```python
from build123d import *

# Parameters (mm, degrees)
SKETCH_W     = 32
SKETCH_H     = 17
PAD_DEPTH    = 1.5
SKETCH001_W  = 6
SKETCH001_H  = 6
PAD001_DEPTH = 2
SKETCH002_R  = 2.710161
PAD002_DEPTH = 7
SKETCH003_W  = 20
SKETCH003_H  = 12
PAD003_DEPTH = 4


with BuildPart() as part:
    # Sketch → Pad (new body)
    with BuildSketch(Plane.XZ):
        with Locations((16, 8.5)):
            Rectangle(SKETCH_W, SKETCH_H)
    extrude(amount=PAD_DEPTH)

    # Sketch001 (on Face4 of Pad) → Pad001 (join)
    with BuildSketch(Plane(origin=(0, 0, 0), x_dir=(0, 0, -1), z_dir=(-1, 0, 0))):
        with Locations((-8.5, 1)):
            Rectangle(SKETCH001_W, SKETCH001_H)
    extrude(amount=PAD001_DEPTH)

    # Sketch002 (on Face13 of Pad001) → Pad002 (join)
    with BuildSketch(Plane(origin=(-2, 0, 0), x_dir=(0, 0, -1), z_dir=(-1, 0, 0))):
        with Locations((-8.5, 1)):
            Circle(SKETCH002_R)
    extrude(amount=PAD002_DEPTH)

    # Sketch003 (on Face5 of Pad002) → Pad003 (join)
    with BuildSketch(Plane.XZ.offset(1.5)):
        with Locations((40, 9)):
            Rectangle(SKETCH003_W, SKETCH003_H)
    extrude(amount=PAD003_DEPTH)


solid = part.part
```
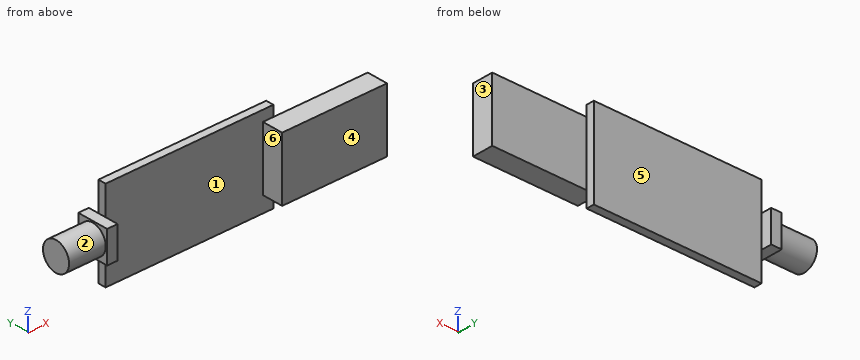
Source: CAD feature listing. Evaluate the final solid. Frame: model axes, mm. Face numbers are marked on the shaded views. A direction names the side the tool comes from. Round coordinates to 2 decimals unless told otherwise and drop trailing zeros. Loops run counter-clockwise (first coordinate to the right, second up) from the corner with the lowest first, then second, coordinate; pieces in that order, holes last. Notation, with made-up numbers: (69, -35.5) - (104, -35.5) arc R21 ccw to (104, -17.5) - close; hole circle Ø2 at (20, 52). An arc over 180 degrees is marked (long way). Use CSV: the item, a comma, the result in double quotes.
Q1. Section query A-A, the plane y = -1. Output: boundary loops of the cut face in (x, z), then the cut area to 3 significant figures.
Reported:
outline,"(-9, 5.79) - (-2, 5.79) - (-2, 5.5) - (0, 5.5) - (0, 0) - (32, 0) - (32, 17) - (0, 17) - (0, 11.5) - (-2, 11.5) - (-2, 11.21) - (-9, 11.21) - close"
area,"594 mm^2"
Q2. Mould query, pull axis X, two halves, no side actions, for the marked faces 1, 2 and 3. Classes: pulls with the +X half, pulls with the -X half, needs draft (parallel to the pull), parting line crosses it, or undercut.
Reported:
face 1,"undercut"
face 2,"needs draft"
face 3,"pulls with the +X half"
Q3. Section query D-D, the plane z = 8.5. Output: boundary loops of the cut face in (x, y), then the cut area to 3 significant figures.
Reported:
outline,"(-9, -3.71) - (-2, -3.71) - (-2, -4) - (0, -4) - (0, -1.5) - (30, -1.5) - (30, -5.5) - (50, -5.5) - (50, -1.5) - (32, -1.5) - (32, 0) - (0, 0) - (0, 2) - (-2, 2) - (-2, 1.71) - (-9, 1.71) - close"
area,"178 mm^2"
Q4. Pin query (flat end, axial travel): pin 1 Ø5 at (x, z) = (9.5, 6.5) entering from +Y; pin 2 Ø4.5 at (x, y) = (41, -2.5) entering from -Z; pin 3 Ø1.2 at (x, y) = (42.5, -3.5) entering from +Z; pin 4 Ø1.5 at (x, y) = (37.5, 1) entering from +Z. Return the tip coordinate at first contact, or that it passes through.
Reported:
pin 1,"y = 0"
pin 2,"z = 3"
pin 3,"z = 15"
pin 4,"through"
Q5. Reachability of the marked faces 4, 5 and 6 from +Z, -Z, +X, -X, +Y, -Y: full face, straight path, thin tool, end or side. Return the list, or none.
Reported:
face 4,"+Z, -Z, +X, -X, -Y"
face 5,"+Z, -Z, +X, +Y"
face 6,"+Z, -Z, -Y"
Q6. Ray query, line 1 along X through (y, z) = (-2.25, 9.5); line 2 along Y through (x, z) = (32.5, 12.25); line 3 along Y through (x, z) = (25, 14). Return the intervals inside material, ascending.
Reported:
line 1,"-9 to 0, 30 to 50"
line 2,"-5.5 to -1.5"
line 3,"-1.5 to 0"
Q7. Section query C-C, the plane x = 18. Output: boundary loops of the cut face in (y, z).
Reported:
outline,"(-1.5, 0) - (0, 0) - (0, 17) - (-1.5, 17) - close"
Q8. Section query B-B, the plane z = 12. Output: boundary loops of the cut face in (x, y), then the cut area to 3 significant figures.
Reported:
outline,"(0, -1.5) - (30, -1.5) - (30, -5.5) - (50, -5.5) - (50, -1.5) - (32, -1.5) - (32, 0) - (0, 0) - close"
area,"128 mm^2"
